Autodesk Inventor part; units mm, degrees
ref_plane "YZ Plane" through (0, 0, 0) normal (1, 0, 0) x (0, 1, 0)
ref_plane "XZ Plane" through (0, 0, 0) normal (0, 1, 0) x (-1, 0, 0)
ref_plane "XY Plane" through (0, 0, 0) normal (0, 0, 1) x (1, 0, 0)
sketch "スケッチ1" plane through (0, 0, 0) normal (0, 0, 1) x (1, 0, 0)
  line L0 (0, 2.5) -> (1.5, 2.5)
  line L1 (1.5, 2.5) -> (1.5, 4)
  line L2 (1.5, 4) -> (3, 4)
  line L3 (3, 4) -> (3, 1.5)
  line L4 (3, 1.5) -> (-0.0006, 1.5)
  line L5 (0, -0.8) -> (0, 4.8) construction
  line L6 (0, 2.5) -> (-1.5, 2.5)
  line L7 (-1.5, 2.5) -> (-1.5, 4)
  line L8 (-1.5, 4) -> (-3, 4)
  line L9 (-3, 4) -> (-3, 1.5)
  line L10 (-3, 1.5) -> (0.0006, 1.5)
  line L11 (-4.2, 0) -> (4.2, 0)
  point P0 (0, 0)
  point P1 (-0.0006, 1.5)
  dimension "d0" = 1.5
  dimension "d1" = 2.5
  dimension "d2" = 1.5
  dimension "d3" = 1.5
  dimension "d4" = 1.5
revolve "回転1" add sketch "スケッチ1" angle 360 about axis through (-10, 0, 0) along (1, 0, 0)
properties part number "Pulley_D3_P6"
Could you check a few things on this model? Use its own coordinates, in mm. A direction names the side the tool comes from. Give positions to 0.01 mm unless a question says otherwise; leave off trailing zeros. Order: outer loops, then holes, each group sorted by start corner. A loop starts at its lowest first (then second) coordinate and runs counter-clockwise, first axis right, second up. Notation, with made-up numbers: (-36.75, -36) - (-6.75, -36) arc R17 ccw to (-6.75, -16) - close; hole circle Ø7 at (-15.75, 52). An arc over 180 degrees is marked (long way). One line per item, written item: value. Start each with the question number.
1. For faces 4 (the face through (1.5, 2, 2)), 5 (the face through (-2.26, -0.867, 3.905)), which set-ups out of +Z, -Z, +X, -X, +Y, -Y let a thin tool reach every point of the face, with its end or its side?
2. Thinking about a two-plate mould opening in X: for faces 1 (the face through (0.02, -0.54, -2.44)), 2 (the face through (3, 2, 0)), 3 (the face through (-3, 2, 0)), which applies, +X half, -X half, draft (parallel to the pull), parting line (faces both ways), or undercut?
3. Imagine slicing it at B-B on y = 0. List the corners of the cut face in (x, z) for me, plus the area to 3 significant figures.
4. For P1, Ø2, axis at x = 2, z = -3, coming from the +Y side; P2, Ø2.5, axis at y = 0, z = 0, coming from the -X side, each with a flat end and sliding along its axis, tell me the tip position at first contact or that it passes through.
5. Imagine slicing it at A-A on z = -2.75. List the corners of the cut face in (x, y) for me, plus the area to 3 significant figures.
6. Imagine slicing it at D-D on y = -1.75. List the corners of the cut face in (x, z) for me, plus the area to 3 significant figures.
7. If I drill on probe 1 along Z at (x, y) = (-0.4, 0); probe 2 along X at (y, z) = (3.25, 1.25); probe 3 along Z at (x, y) = (0.75, -2), over which ranges is the centre line in solid material (lowest first)?
8. Imagine slicing it at C-C on x = 1.1. List the corners of the cut face in (y, z) for me, plus the area to 3 significant figures.
Values:
1. face 4: none
1. face 5: +X, -X
2. face 1: undercut
2. face 2: +X half
2. face 3: -X half
3. outline: (-3, -4) - (-1.5, -4) - (-1.5, -2.5) - (1.5, -2.5) - (1.5, -4) - (3, -4) - (3, -1.5) - (-3, -1.5) - close; (-3, 1.5) - (3, 1.5) - (3, 4) - (1.5, 4) - (1.5, 2.5) - (-1.5, 2.5) - (-1.5, 4) - (-3, 4) - close
3. area: 21.0 mm²
4. P1: y = 3.46
4. P2: through
5. outline: (-3, -2.9) - (-1.5, -2.9) - (-1.5, 2.9) - (-3, 2.9) - close; (1.5, -2.9) - (3, -2.9) - (3, 2.9) - (1.5, 2.9) - close
5. area: 17.4 mm²
6. outline: (-3, -3.6) - (-1.5, -3.6) - (-1.5, -1.79) - (1.5, -1.79) - (1.5, -3.6) - (3, -3.6) - (3, 3.6) - (1.5, 3.6) - (1.5, 1.79) - (-1.5, 1.79) - (-1.5, 3.6) - (-3, 3.6) - close
6. area: 32.3 mm²
7. probe 1: -2.5 to -1.5, 1.5 to 2.5
7. probe 2: -3 to -1.5, 1.5 to 3
7. probe 3: -1.5 to 1.5
8. outline: circle Ø5 at (0, 0); hole circle Ø3 at (0, 0)
8. area: 12.6 mm²
